```python
from build123d import *

# Parameters (mm, degrees)
F0_W     = 115.3964325786
F0_H     = 90.326808393
F1_DEPTH = 50.8
F2_W     = 39.7604890168
F2_H     = 12.6452748664
F3_DEPTH = 90.327808393
F4_W     = 41.0910267383
F4_H     = 18.6301916838
F5_DEPTH = 50.801
F6_R     = 3.3975971179
F6_W     = 27.4064959049
F6_H     = 7.1375382304
F7_DEPTH = 115.3974325786


with BuildPart() as f1:
    # F0 (on Top) → F1 (new body)
    with BuildSketch(Plane.XY):
        Rectangle(F0_W, F0_H)
    extrude(amount=F1_DEPTH)

    # F2 (on face) → F3 (cut, through all)
    with BuildSketch(Plane.XZ.offset(45.1634041965)):
        Polygon((57.6982162893, 50.8), (0, 50.8), (57.6982162893, 0), align=None)
        with Locations((-37.8179717809, 6.3226374332)):
            Rectangle(F2_W, F2_H)
    extrude(amount=-F3_DEPTH, mode=Mode.SUBTRACT)

    # F4 (on face) → F5 (cut, through all)
    with BuildSketch(Plane(origin=(0, 0, 0), x_dir=(1, 0, 0), z_dir=(0, 0, -1))):
        with Locations((37.1527029201, 35.8483083546)):
            Rectangle(F4_W, F4_H)
    extrude(amount=-F5_DEPTH, mode=Mode.SUBTRACT)

    # F6 (on face) → F7 (cut, through all)
    with BuildSketch(Plane(origin=(-57.6982162893, 0, 0), x_dir=(0, -1, 0), z_dir=(-1, 0, 0))):
        with Locations((-20.8592172712, 21.3062018156)):
            Circle(F6_R)
        with Locations((-20.8592191339, 32.9277664423)):
            Circle(F6_R)
        with Locations((5.6617897935, 32.9277664423)):
            Circle(F6_R)
        with Locations((5.065811798, 21.008213982)):
            Circle(F6_R)
        with Locations((-6.5557556227, 47.2312308848)):
            Rectangle(F6_W, F6_H)
    extrude(amount=-F7_DEPTH, mode=Mode.SUBTRACT)


solid = f1.part
```
CAD build for the part. Positions are in the model's coordinates, mm. A direction names the side the tool comes from. Give positions to 0.01 mm unless a question says otherwise; leave off trailing zeros. Loops run counter-clockwise (first coordinate to the right, second up) from the corner with the lowest first, then second, coordinate; pieces in that order, holes last. Notation, with made-up numbers: M -13.75,-35.75 L -4.75,-35.75 A26 ccw -4.75,-19.75 Z; hole C -26.5,75 d8. An arc over 180 degrees is marked long. Use one line per item in the form item = value.
Item 1: Flat gauge pins, fed straight in: pin 1 (6 mm diameter, centred on x = 13.5, y = 6, fed in from +Z); pin 2 (5 mm diameter, centred on x = -39, y = 12, fed in from +Z); pin 3 (8 mm diameter, centred on y = 20.86, z = 32.93, fed in from +X). Where does each tip first touch, or does it go through?
Determined:
pin_1 = 41.56
pin_2 = 43.66
pin_3 = 24.84
Item 2: Two-plate mould, pull along Y, no slides. Class faces 6 (the face through (28.445, 9.404, 25.756)), 7 (the face through (-17.3, -4.93, 29.61)), 8 (the face through (32, -26.533, 14)), 9 (the face through (-10.6, -4.3, 17.7)): pulls with the +Y half, pulls with the -Y half, needs draft (parallel to the pull), parting line crosses it, or undercut.
Determined:
face_6 = needs draft
face_7 = undercut
face_8 = pulls with the -Y half
face_9 = undercut
Item 3: Slice it at B-B (x = -2.5). List the corners of the cut face in (y, z).
Determined:
outline = M -45.16,0 L 45.16,0 L 45.16,50.8 L 20.26,50.8 L 20.26,43.66 L -7.15,43.66 L -7.15,50.8 L -45.16,50.8 Z; hole C -5.66,32.93 d6.8; hole C -5.07,21.01 d6.8; hole C 20.86,21.31 d6.8; hole C 20.86,32.93 d6.8
Item 4: Which spindle directions (+Z, -Z, +X, -X, +Y, -Y) get a long thin tool onto all of the face, cutting with end or side? Do faces 1 (the face through (-14, 45.163, 25)), 2 (the face through (-10.79, 21.6, 17.99)), 3 (the face through (-17.938, -1, 6)), 4 (the face through (-25, -7.147, 47)), 5 (the face through (16.607, -36, 18)). Say none if no direction does.
Determined:
face_1 = +Z, -Z, +X, -X, +Y
face_2 = +X, -X
face_3 = -Z, -X, +Y, -Y
face_4 = +Z, +X, -X
face_5 = +Z, -Z, +X, -Y
Item 5: Slice it at C-C (y = -34.5). List the corners of the cut face in (x, z), plus the area to 3 significant figures.
Determined:
outline = M -57.7,12.65 L -17.94,12.65 L -17.94,0 L 16.61,0 L 16.61,36.18 L 0,50.8 L -57.7,50.8 Z
area = 3,150 mm2
Item 6: Drill centre lines: probe 1 along Y at (x, z) = (0, 23); probe 2 along Y at (x, z) = (-14, 33.5); probe 3 along Z at (x, y) = (-45, 38.5). Where is each one in solid material? Low to high. Write a range as from..to.
Determined:
probe_1 = -45.16..-7.82, -2.31..17.91, 23.8..45.16
probe_2 = -45.16..-9.01, -2.31..17.51, 24.21..45.16
probe_3 = 12.65..50.8
Item 7: Slice it at A-A (z = 45). List the corners of the cut face in (x, y).
Determined:
outline = M -57.7,-45.16 L 6.59,-45.16 L 6.59,-7.15 L -57.7,-7.15 Z; M -57.7,20.26 L 6.59,20.26 L 6.59,45.16 L -57.7,45.16 Z
Item 8: Slice it at D-D (z = 26). List the corners of the cut face in (x, y).
Determined:
outline = M -57.7,-45.16 L 16.61,-45.16 L 16.61,-26.53 L 28.17,-26.53 L 28.17,45.16 L -57.7,45.16 Z
